Can you work these out from the model? Positions are in its coordinate system, mm. A direction names the side the tool comes from. Coordinates: 2 decimals unless noted, no trailing zeros. Loops run counter-clockwise (first coordinate to the right, second up) from the corner with the lowest first, then second, coordinate; pieces in that order, holes last. Notation, with made-up numbers: (11.5, 6) -> (25.5, 6) arc R17 cw to (25.5, 13) -> close; hole circle Ø1 at (65.25, 38). An arc over 180 degrees is marked (long way). Put each result on its own line as item: value. Start each with the question number.
Item 1: For faces 1 (the flat face through (-0.11, 1.52, -0.73)), 2 (the flat face through (0, 3, 0)), 3 (the flat face through (23, 5, 0)), which set-ups out of +Z, -Z, +X, -X, +Y, -Y let a thin tool reach every point of the face, with its end or its side?
Item 2: We'd pull the mould along Z, two halves only. Please class faces 4 (the cylindrical face through (21.797, 5.07, -15.359)), 5 (the flat face through (-8, 2, -4)), 6 (the flat face through (-2.74, 1.52, -1.28)), 7 (the flat face through (5, 5, 19)): pulls with the +Z half, pulls with the -Z half, needs draft (parallel to the pull), parting line crosses it, or undercut.
Item 3: If we section it at B-B on y = 7: Please give me the cut outline in (x, z).
Item 4: If we section it at C-C on z = 21.5: Please give me the cut outline in (x, y), plus the area to 3 significant figures.
Item 5: If we section it at A-A on x = 11: Please give me the cut outline in (y, z), plus the area to 3 significant figures.
Item 6: Please list where these lines run through material, in increasing order: L1, parallel to Z at x = 13, y = 1.25; L2, parallel to Z at x = -10, y = 7.5; L3, parallel to X at y = 6.25, z = -21.5. Write a range as from..to.
Item 7: Will these pins go through, and if not, where does the flat tip stop? P1, Ø5, axis at x = 14, z = 3, coming from the -Y side; P2, Ø1.5, axis at x = 4.5, y = 1.5, coming from the +Z side; P3, Ø1, axis at x = -2.5, y = 1, coming from the -Z side; P4, Ø1.4, axis at x = -2.5, y = 1, coming from the +Z side.
Item 8: If we section it at D-D on x = -12: Please give me the cut outline in (y, z).
```python
from build123d import *

# Parameters (mm, degrees)
BASE_W               = 46
BASE_H               = 33
SHELL_DEPTH          = 10
SHELLHOLE_W          = 41
SHELLHOLE_H          = 28
HOLE_DEPTH           = 7
PINHOLES_W           = 23
PINHOLES_H           = 4
PINS_DEPTH           = 3
SKETCH10_W           = 10
SKETCH10_H           = 10
BOSS_EXTRUDE3_DEPTH  = 10
SKETCH11_R           = 2
CUT_EXTRUDE3_DEPTH   = 10
FILLET1_R            = 4
FILLET1_OF_MIRROR1_R = 4
FILLET2_R            = 4
AIR1_DEPTH           = 10


with BuildPart() as part:
    # Base → Shell (new body)
    with BuildSketch(Plane(origin=(0, 0, 0), x_dir=(1, 0, 0), z_dir=(0, 1, 0))):
        Rectangle(BASE_W, BASE_H)
    extrude(amount=SHELL_DEPTH)

    # ShellHole → Hole (cut)
    with BuildSketch(Plane(origin=(0, 10, 0), x_dir=(1, 0, 0), z_dir=(0, 1, 0))):
        Rectangle(SHELLHOLE_W, SHELLHOLE_H)
    extrude(amount=-HOLE_DEPTH, mode=Mode.SUBTRACT)

    # PinHoles → Pins (cut)
    with BuildSketch(Plane(origin=(0, 0, 0), x_dir=(-1, 0, 0), z_dir=(0, -1, 0))):
        with Locations((-5.8, -11.5)):
            Rectangle(PINHOLES_W, PINHOLES_H)
        with Locations((-5.8, 11.5)):
            Rectangle(PINHOLES_W, PINHOLES_H)
    extrude(amount=-PINS_DEPTH, mode=Mode.SUBTRACT)

    # Sketch10 → Boss-Extrude3 (add)
    with BuildSketch(Plane.XY.offset(16.5)):
        with Locations((0, 5)):
            Rectangle(SKETCH10_W, SKETCH10_H)
    boss_extrude3 = extrude(amount=BOSS_EXTRUDE3_DEPTH)

    # Sketch11 → Cut-Extrude3 (cut)
    with BuildSketch(Plane(origin=(0, 10, 0), x_dir=(1, 0, 0), z_dir=(0, 1, 0))):
        with Locations(Location((0, -21.5, 0), (0, 0, 270))):
            Circle(SKETCH11_R)
    cut_extrude3 = extrude(amount=-CUT_EXTRUDE3_DEPTH, mode=Mode.SUBTRACT)

    # Fillet1
    fillet1_edges = [part.edges().sort_by_distance(p)[0] for p in [
        (5, 5, 26.5),
        (-5, 5, 26.5),
    ]]
    fillet(fillet1_edges, radius=FILLET1_R)

    # Mirror1: Boss-Extrude3, Cut-Extrude3 across plane
    add(boss_extrude3.mirror(Plane.XY))
    add(cut_extrude3.mirror(Plane.XY), mode=Mode.SUBTRACT)

    # Fillet1 of Mirror1
    fillet1_of_mirror1_edges = [part.edges().sort_by_distance(p)[0] for p in [
        (5, 5, -26.5),
        (-5, 5, -26.5),
    ]]
    fillet(fillet1_of_mirror1_edges, radius=FILLET1_OF_MIRROR1_R)

    # Fillet2
    fillet2_edges = [part.edges().sort_by_distance(p)[0] for p in [
        (-23, 5, -16.5),
        (23, 5, -16.5),
        (23, 5, 16.5),
        (-23, 5, 16.5),
    ]]
    fillet(fillet2_edges, radius=FILLET2_R)

    # AirHole → Air1 (cut)
    with BuildSketch(Plane(origin=(0, 3, 0), x_dir=(1, 0, 0), z_dir=(0, 1, 0))):
        Polygon((-3.5, 2.598076211), (-6.5, 2.598076211), (-8, 0), (-6.5, -2.598076211), (-3.5, -2.598076211), (-2, 0), align=None)
        Polygon((-10.214101615, 4.165063509), (-8.482050808, 3.165063509), (-7.654700538, 4.598076211), (-6, 4.598076211), (-6, 6.598076211), (-8.809401077, 6.598076211), align=None)
        Polygon((-11.214101615, -2.433012702), (-9.482050808, -1.433012702), (-10.309401077, 0), (-9.482050808, 1.433012702), (-11.214101615, 2.433012702), (-12.618802154, 0), align=None)
        Polygon((-7.654700538, -4.598076211), (-8.482050808, -3.165063509), (-10.214101615, -4.165063509), (-8.809401077, -6.598076211), (-6, -6.598076211), (-6, -4.598076211), align=None)
        Polygon((-2.345299462, -4.598076211), (-4, -4.598076211), (-4, -6.598076211), (-1.190598923, -6.598076211), (0.214101615, -4.165063509), (-1.517949192, -3.165063509), align=None)
        Polygon((0.309401077, 0), (-0.517949192, -1.433012702), (1.214101615, -2.433012702), (2.618802154, 0), (1.214101615, 2.433012702), (-0.517949192, 1.433012702), align=None)
        Polygon((-4, 6.598076211), (-4, 4.598076211), (-2.345299462, 4.598076211), (-1.517949192, 3.165063509), (0.214101615, 4.165063509), (-1.190598923, 6.598076211), align=None)
    extrude(amount=-AIR1_DEPTH, mode=Mode.SUBTRACT)


solid = part.part
```
Solutions:
1. face 1: +Y, -Y
1. face 2: +Y
1. face 3: +Z, -Z, +X, +Y, -Y
2. face 4: pulls with the -Z half
2. face 5: undercut
2. face 6: undercut
2. face 7: needs draft
3. outline: (-23, -12.5) arc R4 ccw to (-19, -16.5) -> (-5, -16.5) -> (-5, -22.5) arc R4 ccw to (-1, -26.5) -> (1, -26.5) arc R4 ccw to (5, -22.5) -> (5, -16.5) -> (19, -16.5) arc R4 ccw to (23, -12.5) -> (23, 12.5) arc R4 ccw to (19, 16.5) -> (5, 16.5) -> (5, 22.5) arc R4 ccw to (1, 26.5) -> (-1, 26.5) arc R4 ccw to (-5, 22.5) -> (-5, 16.5) -> (-19, 16.5) arc R4 ccw to (-23, 12.5) -> close; hole (-20.5, -14) -> (20.5, -14) -> (20.5, 14) -> (-20.5, 14) -> close; hole circle Ø4 at (0, -21.5); hole circle Ø4 at (0, 21.5)
4. outline: (-5, 0) -> (-2, 0) -> (-2, 10) -> (-5, 10) -> close; (2, 0) -> (5, 0) -> (5, 10) -> (2, 10) -> close
4. area: 60.0 mm^2
5. outline: (0, -16.5) -> (10, -16.5) -> (10, -14) -> (3, -14) -> (3, -13.5) -> (0, -13.5) -> close; (0, -9.5) -> (3, -9.5) -> (3, 9.5) -> (0, 9.5) -> close; (0, 13.5) -> (3, 13.5) -> (3, 14) -> (10, 14) -> (10, 16.5) -> (0, 16.5) -> close
5. area: 110 mm^2
6. L1: -16.5..-13.5, -9.5..9.5, 13.5..16.5
6. L2: -16.5..-14, 14..16.5
6. L3: -5..-2, 2..5
7. P1: y = 0
7. P2: z = 25.4
7. P3: z = -26.37
7. P4: z = 26.42
8. outline: (0, -16.5) -> (10, -16.5) -> (10, -14) -> (3, -14) -> (3, -1.07) -> (0, -1.07) -> close; (0, 1.07) -> (3, 1.07) -> (3, 14) -> (10, 14) -> (10, 16.5) -> (0, 16.5) -> close
